Build history of the part. All positions in model axes, mm. Round coordinates to 2 decimals unless told otherwise and drop trailing zeros. Order: outer loops, then holes, each group sorted by start corner. A loop starts at its lowest first (then second) coordinate and runs counter-clockwise, first axis right, second up. Notation, with made-up numbers: (50.5, -20.75) -> (89.5, -20.75) arc R22 cw to (89.5, -3.75) -> close; hole circle Ø6 at (59, 11). An arc over 180 degrees is marked (long way). Answer as a JSON object with one key per item and string values.
from build123d import *

# Parameters (mm, degrees)
SKETCH_W  = 13
SKETCH_H  = 18
SKETCH_R  = 0.95
PAD_DEPTH = 7


with BuildPart() as part:
    # Sketch → Pad (new body)
    with BuildSketch(Plane.YZ):
        with Locations((6.5, 9)):
            Rectangle(SKETCH_W, SKETCH_H)
        with Locations((1.42, 16.62)):
            Circle(SKETCH_R, mode=Mode.SUBTRACT)
        with Locations((11.58, 16.62)):
            Circle(SKETCH_R, mode=Mode.SUBTRACT)
        with Locations((11.58, 1.38)):
            Circle(SKETCH_R, mode=Mode.SUBTRACT)
        with Locations((3.96, 16.62)):
            Circle(SKETCH_R, mode=Mode.SUBTRACT)
        with Locations((6.5, 16.62)):
            Circle(SKETCH_R, mode=Mode.SUBTRACT)
        with Locations((9.04, 16.62)):
            Circle(SKETCH_R, mode=Mode.SUBTRACT)
        with Locations((11.58, 6.46)):
            Circle(SKETCH_R, mode=Mode.SUBTRACT)
        with Locations((11.58, 9)):
            Circle(SKETCH_R, mode=Mode.SUBTRACT)
        with Locations((11.58, 11.54)):
            Circle(SKETCH_R, mode=Mode.SUBTRACT)
        with Locations((11.58, 14.08)):
            Circle(SKETCH_R, mode=Mode.SUBTRACT)
        with Locations((11.58, 3.92)):
            Circle(SKETCH_R, mode=Mode.SUBTRACT)
        with Locations((9.04, 14.08)):
            Circle(SKETCH_R, mode=Mode.SUBTRACT)
        with Locations((6.5, 14.08)):
            Circle(SKETCH_R, mode=Mode.SUBTRACT)
        with Locations((3.96, 14.08)):
            Circle(SKETCH_R, mode=Mode.SUBTRACT)
        with Locations((1.42, 14.08)):
            Circle(SKETCH_R, mode=Mode.SUBTRACT)
        with Locations((9.04, 11.54)):
            Circle(SKETCH_R, mode=Mode.SUBTRACT)
        with Locations((6.5, 11.54)):
            Circle(SKETCH_R, mode=Mode.SUBTRACT)
        with Locations((3.96, 11.54)):
            Circle(SKETCH_R, mode=Mode.SUBTRACT)
        with Locations((1.42, 11.54)):
            Circle(SKETCH_R, mode=Mode.SUBTRACT)
        with Locations((9.04, 9)):
            Circle(SKETCH_R, mode=Mode.SUBTRACT)
        with Locations((6.5, 9)):
            Circle(SKETCH_R, mode=Mode.SUBTRACT)
        with Locations((3.96, 9)):
            Circle(SKETCH_R, mode=Mode.SUBTRACT)
        with Locations((1.42, 9)):
            Circle(SKETCH_R, mode=Mode.SUBTRACT)
        with Locations((9.04, 6.46)):
            Circle(SKETCH_R, mode=Mode.SUBTRACT)
        with Locations((6.5, 6.46)):
            Circle(SKETCH_R, mode=Mode.SUBTRACT)
        with Locations((3.96, 6.46)):
            Circle(SKETCH_R, mode=Mode.SUBTRACT)
        with Locations((1.42, 6.46)):
            Circle(SKETCH_R, mode=Mode.SUBTRACT)
        with Locations((1.42, 3.92)):
            Circle(SKETCH_R, mode=Mode.SUBTRACT)
        with Locations((3.96, 3.92)):
            Circle(SKETCH_R, mode=Mode.SUBTRACT)
        with Locations((6.5, 3.92)):
            Circle(SKETCH_R, mode=Mode.SUBTRACT)
        with Locations((9.04, 3.92)):
            Circle(SKETCH_R, mode=Mode.SUBTRACT)
        with Locations((9.04, 1.38)):
            Circle(SKETCH_R, mode=Mode.SUBTRACT)
        with Locations((6.5, 1.38)):
            Circle(SKETCH_R, mode=Mode.SUBTRACT)
        with Locations((3.96, 1.38)):
            Circle(SKETCH_R, mode=Mode.SUBTRACT)
        with Locations((1.42, 1.38)):
            Circle(SKETCH_R, mode=Mode.SUBTRACT)
    extrude(amount=PAD_DEPTH)


solid = part.part
1) Probe L1, parallel to Y at x = 5.75, z = 4; L2, parallel to Y at x = 3.25, z = 17. List the from-to ranges inside material, lowest first. Write a range as from..to.
Checked values:
{"L1": "y = 0..0.47, 2.37..3.01, 4.91..5.55, 7.45..8.09, 9.99..10.63, 12.53..13", "L2": "y = 0..0.55, 2.29..3.09, 4.83..5.63, 7.37..8.17, 9.91..10.71, 12.45..13"}
2) Cut at A-A, the plane y = 9.04. Count the separate pieces of the cut face and the enclosed holes in it, plus the area to 3 significant figures.
Checked values:
{"separate pieces": "8", "enclosed holes": "0", "area": "32.9 mm²"}
3) Pull direction Z, two halves, no side cores. Call faces 1 (the face through (3.45, 8.34, 2.02)), 2 (the face through (3, 0, 9)), 3 (the face through (3, 6, 18)): pulls with the +Z half, pulls with the -Z half, needs draft (parallel to the pull), parting line crosses it, or undercut.
Checked values:
{"face 1": "undercut", "face 2": "needs draft", "face 3": "pulls with the +Z half"}
4) Cut at C-C, the plane z = 3.25. Give the cut face in (x, y), plus the area to 3 significant figures.
Checked values:
{"outline": "(0, 0) -> (7, 0) -> (7, 0.75) -> (0, 0.75) -> close; (0, 2.09) -> (7, 2.09) -> (7, 3.29) -> (0, 3.29) -> close; (0, 4.63) -> (7, 4.63) -> (7, 5.83) -> (0, 5.83) -> close; (0, 7.17) -> (7, 7.17) -> (7, 8.37) -> (0, 8.37) -> close; (0, 9.71) -> (7, 9.71) -> (7, 10.91) -> (0, 10.91) -> close; (0, 12.25) -> (7, 12.25) -> (7, 13) -> (0, 13) -> close", "area": "43.9 mm²"}
5) Cut at B-B, the plane z = 9. Give the cut face in (x, y), plus the area to 3 significant figures.
Checked values:
{"outline": "(0, 0) -> (7, 0) -> (7, 0.47) -> (0, 0.47) -> close; (0, 2.37) -> (7, 2.37) -> (7, 3.01) -> (0, 3.01) -> close; (0, 4.91) -> (7, 4.91) -> (7, 5.55) -> (0, 5.55) -> close; (0, 7.45) -> (7, 7.45) -> (7, 8.09) -> (0, 8.09) -> close; (0, 9.99) -> (7, 9.99) -> (7, 10.63) -> (0, 10.63) -> close; (0, 12.53) -> (7, 12.53) -> (7, 13) -> (0, 13) -> close", "area": "24.5 mm²"}
